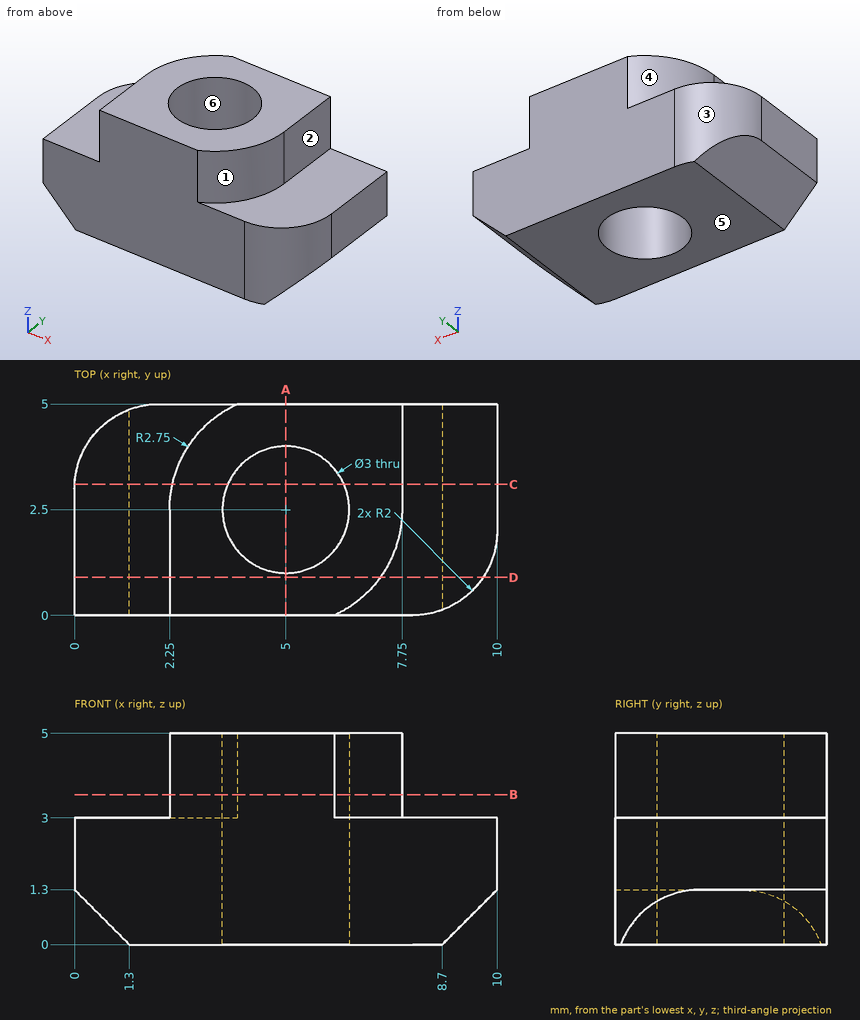
Geometry check sheet. Reference: drawing and pictorial views, mm from the part's lowest x, y, z. A direction names the side the tool comes from. Round coordinates to 2 decimals unless told otherwise and drop trailing zeros. Loops run counter-clockwise (first coordinate to the right, second up) from the corner with the lowest first, then second, coordinate; pieces in that order, holes last. Notation, with made-up numbers: (4, -34.75) - (49, -34.75) arc R24 cw to (49, 3.25) - close; hole circle Ø6 at (29, 33.5). An arc over 180 degrees is marked (long way). Answer as CSV lines item,"result".
(1) Material ranges on line 1 along Y through (x, z) = (5, 1.75); line 2 along Y through (x, z) = (5.5, 1.8); line 3 along X through (y, z) = (3.6, 3.9), recorded low to high.
Output values:
line 1,"y = 0 to 1, 4 to 5"
line 2,"y = 0 to 1.09, 3.91 to 5"
line 3,"x = 2.48 to 3.98, 6.02 to 7.75"
(2) Cross-section at D-D, the plane y = 0.9. Enter the section's corners in (x, z).
Output values:
outline,"(0, 1.3) - (1.3, 0) - (8.7, 0) - (9.67, 0.97) - (9.67, 3) - (7.24, 3) - (7.24, 5) - (2.25, 5) - (2.25, 3) - (0, 3) - close"
(3) Depth check by flat-ended pin: pin 1 Ø1.2 at (x, y) = (9, 2.5) entering from +Z; pin 2 Ø1 at (y, z) = (3.5, 4.5) entering from +X; pin 3 Ø2.5 at (x, y) = (5, 2.5) entering from +Z. Enter the tip coordinate at first touch or a pass-through.
Output values:
pin 1,"stops at z = 3"
pin 2,"stops at x = 7.75"
pin 3,"passes through"
(4) Cross-section at C-C, the plane y = 3.1. Enter the section's corners in (x, z).
Output values:
outline,"(0, 1.3) - (1.3, 0) - (3.63, 0) - (3.63, 5) - (2.32, 5) - (2.32, 3) - (0, 3) - close; (6.37, 0) - (8.7, 0) - (10, 1.3) - (10, 3) - (7.75, 3) - (7.75, 5) - (6.37, 5) - close"
(5) Set-up check for the marked faces 1, 2 and 3: record each of +Z, -Z, +X, -X, +Y, -Y from which the full face is reachable in a straight line by a thin tool's end or side.
Output values:
face 1,"+Z, +X, -Y"
face 2,"+Z, +X, +Y, -Y"
face 3,"+Z, -Z, -X, +Y"
(6) Cross-section at A-A, the plane x = 5. Enter the section's corners in (y, z), and give its area (3 significant figures).
Output values:
outline,"(0, 0) - (1, 0) - (1, 5) - (0, 5) - close; (4, 0) - (5, 0) - (5, 5) - (4, 5) - close"
area,"10.0 mm²"
(7) Cross-section at B-B, the plane z = 3.55. Enter the section's corners in (x, y), and give its area (3 significant figures).
Output values:
outline,"(2.25, 0) - (6.15, 0) arc R2.75 ccw to (7.75, 2.5) - (7.75, 5) - (3.85, 5) arc R2.75 ccw to (2.25, 2.5) - close; hole circle Ø3 at (5, 2.5)"
area,"18.2 mm²"
(8) Release check for a two-part mould opening along Y. For the marked faces 4, 5 and 6 record: released by +Y, released by -Y, zero draft, split by the parting line, or undercut.
Output values:
face 4,"released by +Y"
face 5,"zero draft"
face 6,"undercut"
